from build123d import *

# Parameters (mm, degrees)
BOSS_EXTRUDE1_DEPTH = 7
SKETCH3_R           = 1.25
CUT_EXTRUDE1_DEPTH  = 10


with BuildPart() as part:
    # Sketch2 → Boss-Extrude1 (new body)
    with BuildSketch(Plane.XY):
        with BuildLine():
            Line((-5.004882759, -8.657433139), (-5.004882759, -68.657433139))
            Line((-5.004882759, -68.657433139), (-9.004882759, -68.657433139))
            Line((-9.004882759, -68.657433139), (-9.004882759, -71.657433139))
            Line((-9.004882759, -71.657433139), (-2.004882759, -71.657433139))
            Line((-2.004882759, -71.657433139), (-2.004882759, -9.796961015))
            ThreePointArc((-2.004882759, -9.796961015), (0, -10), (2.004882759, -9.796961015))
            Line((2.004882759, -9.796961015), (2.004882759, -71.657433139))
            Line((2.004882759, -71.657433139), (9.004882759, -71.657433139))
            Line((9.004882759, -71.657433139), (9.004882759, -68.657433139))
            Line((9.004882759, -68.657433139), (5.004882759, -68.657433139))
            Line((5.004882759, -68.657433139), (5.004882759, -8.657433139))
            ThreePointArc((5.004882759, -8.657433139), (8.661663454, -4.997558024), (10, 0))
            Line((10, 0), (7, 0))
            ThreePointArc((7, 0), (0, -7), (-7, 0))
            Line((-7, 0), (-10, 0))
            ThreePointArc((-10, 0), (-8.661663454, -4.997558024), (-5.004882759, -8.657433139))
        make_face()
    extrude(amount=BOSS_EXTRUDE1_DEPTH)

    # Sketch3 → Cut-Extrude1 (cut)
    with BuildSketch(Plane(origin=(0, -68.657433139, 0), x_dir=(1, 0, 0), z_dir=(0, 1, 0))):
        with Locations(Location((-7.084526396, -3.795336707, 0), (0, 0, 270))):
            Circle(SKETCH3_R)
        with Locations(Location((7.239366758, -3.795336707, 0), (0, 0, 270))):
            Circle(SKETCH3_R)
    extrude(amount=-CUT_EXTRUDE1_DEPTH, mode=Mode.SUBTRACT)


solid = part.part
Design review of the part built by this model. Coordinates are the model's own, in mm. A direction names the side the tool comes from. Give positions to 0.01 mm unless a question says otherwise; leave off trailing zeros. Loops run counter-clockwise (first coordinate to the right, second up) from the corner with the lowest first, then second, coordinate; pieces in that order, holes last. Notation, with made-up numbers: (13, 73.25) - (65, 73.25) arc R10 ccw to (65, 80.25) - close; hole circle Ø1 at (-1.75, 78.5). An arc over 180 degrees is marked (long way). Write item = value, one per line.
1) Take a section at A-A on y = -25. State the section outline as (x, z) points.
Result sheet:
outline = (-5, 0) - (-2, 0) - (-2, 7) - (-5, 7) - close; (2, 0) - (5, 0) - (5, 7) - (2, 7) - close
2) Tool access review of faces 4 (the face through (-5.005, -38, 3)), 5 (the face through (-2.005, -41, 3)), 6 (the face through (8.6, -5.1, 3.5)): name each direction out of +Z, -Z, +X, -X, +Y, -Y from which nothing blocks a thin tool from reaching the whole face with its end or side.
Result sheet:
face_4 = +Z, -Z, -X
face_5 = +Z, -Z, -Y
face_6 = +Z, -Z, +X
3) Clearance check with flat-ended pins moving along their axes: pin 1 Ø1.5 at (y, z) = (-22.5, 5) entering from +X; pin 2 Ø2.5 at (y, z) = (-71, 5) entering from -X; pin 3 Ø0.9 at (y, z) = (-70.5, 3) entering from +X. State where each tip first meets the part, or that it passes through.
Result sheet:
pin_1 = 5
pin_2 = -9
pin_3 = 9
4) To check wall thickness, follow line 1 (X direction, y = -12, z = 3.5); line 2 (Y direction, x = -5.5, z = 3.5); line 3 (Y direction, x = 8.75, z = 6.75). State the ranges of each line that lie inside material, in increasing order.
Result sheet:
line_1 = -5 to -2, 2 to 5
line_2 = -71.66 to -68.66, -8.35 to -4.33
line_3 = -71.66 to -68.66, -4.84 to 0
5) Take a section at D-D on x = 4.25. State the section outline as (y, z) points.
Result sheet:
outline = (-71.66, 0) - (-5.56, 0) - (-5.56, 7) - (-71.66, 7) - close
6) Draft analysis for pull direction Z (two halves, no side actions). For faces 1 (the face through (5.005, -39, 3)), 2 (the face through (-2.4, -35.3, 0)), 3 (the face through (-7.845, -70.136, 2.803)), state which applies: +Z half, -Z half, draft (parallel to the pull), parting line (faces both ways), or undercut.
Result sheet:
face_1 = draft
face_2 = -Z half
face_3 = undercut
7) Take a section at C-C on x = 0. State the section outline as (y, z) points.
Result sheet:
outline = (-10, 0) - (-7, 0) - (-7, 7) - (-10, 7) - close
8) Take a section at B-B on z = 3.5. State the section outline as (x, y) points.
Result sheet:
outline = (-10, 0) arc R10 ccw to (-5, -8.66) - (-5, -68.66) - (-5.87, -68.66) - (-5.87, -71.66) - (-2, -71.66) - (-2, -9.8) arc R10 ccw to (2, -9.8) - (2, -71.66) - (6.02, -71.66) - (6.02, -68.66) - (5, -68.66) - (5, -8.66) arc R10 ccw to (10, 0) - (7, 0) arc R7 cw to (-7, 0) - close; (-9, -71.66) - (-8.3, -71.66) - (-8.3, -68.66) - (-9, -68.66) - close; (8.45, -71.66) - (9, -71.66) - (9, -68.66) - (8.45, -68.66) - close
